The listing builds one solid part. Answer for the finished solid, in the listing's coordinates (mm). Round coordinates to 2 decimals unless told otherwise and drop trailing zeros. Write each loop counter-clockwise with the first axis right and the second up, starting at its lowest first coordinate (ties: lowest second). Pieces come first, ordered by that corner, then holes.
Item 1: Find section C-C on z = -77.5. Give the vertices of the cut face in (x, y) (3 decimals).
Item 2: Find section A-A on x = 0. Give the vertices of the cut face in (y, z), then the cut area to 3 significant figures.
Item 3: Find section B-B on z = 0. Give the vertices of the cut face in (x, y).
Item 4: Find the intervals of material crossed by probe 1 along X at (y, z) = (4.25, -77); probe 2 along X at (y, z) = (0.5, 27); probe 3 along Z at (x, y) = (-22.5, 1.75), in increasing order.
Item 5: Find section D-D on x = 65. Give the vertices of the cut face in (y, z) (3 decimals).
Item 6: For a pull along Z with two mould halves and no side action, classify faces 1 (the face through (-39, 0, -1)), 2 (the face through (-26.063, 3.118, 67.626)), 3 (the face through (-1, 3, 85)) as +Z half, -Z half, draft (parallel to the pull), parting line (faces both ways), or undercut.
```python
from build123d import *

# Parameters (mm, degrees)
SKETCH1_W                      = 170
SKETCH1_H                      = 170
SKETCH1_R                      = 32
BOSS_EXTRUDE3_DEPTH            = 6.35
M4_CLEARANCE_HOLE2_D           = 4.5
M4_CLEARANCE_HOLE2_CSINK_D     = 4.55
M4_CLEARANCE_HOLE2_CSINK_ANGLE = 90
M4_CLEARANCE_HOLE5_D           = 4.5
M4_CLEARANCE_HOLE5_CSINK_D     = 4.55
M4_CLEARANCE_HOLE5_CSINK_ANGLE = 90
M5_CLEARANCE_HOLE1_D           = 5.5
M5_CLEARANCE_HOLE1_CSINK_D     = 5.55
M5_CLEARANCE_HOLE1_CSINK_ANGLE = 90
M5_CLEARANCE_HOLE2_D           = 5.5
M5_CLEARANCE_HOLE2_CSINK_D     = 5.55
M5_CLEARANCE_HOLE2_CSINK_ANGLE = 90


with BuildPart() as part:
    # Sketch1 → Boss-Extrude3 (new body)
    with BuildSketch(Plane(origin=(0, 0, 0), x_dir=(1, 0, 0), z_dir=(0, 1, 0))):
        Rectangle(SKETCH1_W, SKETCH1_H)
        with Locations(Location((0, 0, 0), (0, 0, 270))):
            Circle(SKETCH1_R, mode=Mode.SUBTRACT)
    extrude(amount=BOSS_EXTRUDE3_DEPTH)

    # M4 Clearance Hole2 (through all)
    with Locations(Plane(origin=(0, 0, 0), x_dir=(-1, 0, 0), z_dir=(0, -1, 0))):
        with Locations((-9.188076101, 34.290366833), (25.102290732, 25.102290732), (34.290366833, -9.188076101), (9.188076101, -34.290366833), (-25.102290732, -25.102290732), (-34.290366833, 9.188076101)):
            CounterSinkHole(M4_CLEARANCE_HOLE2_D / 2, M4_CLEARANCE_HOLE2_CSINK_D / 2, counter_sink_angle=M4_CLEARANCE_HOLE2_CSINK_ANGLE)

    # M4 Clearance Hole5 (through all)
    with Locations(Plane(origin=(0, 6.35, 0), x_dir=(1, 0, 0), z_dir=(0, 1, 0))):
        with Locations((-68.301673362, -23.916580707), (-23.916580707, -68.301673362)):
            CounterSinkHole(M4_CLEARANCE_HOLE5_D / 2, M4_CLEARANCE_HOLE5_CSINK_D / 2, counter_sink_angle=M4_CLEARANCE_HOLE5_CSINK_ANGLE)

    # M5 Clearance Hole1 (through all)
    with Locations(Plane(origin=(0, 6.35, 0), x_dir=(1, 0, 0), z_dir=(0, 1, 0))):
        with Locations((-65, -77.5)):
            CounterSinkHole(M5_CLEARANCE_HOLE1_D / 2, M5_CLEARANCE_HOLE1_CSINK_D / 2, counter_sink_angle=M5_CLEARANCE_HOLE1_CSINK_ANGLE)

    # M5 Clearance Hole2 (through all)
    with Locations(Plane(origin=(0, 6.35, 0), x_dir=(1, 0, 0), z_dir=(0, 1, 0))):
        with Locations((-65, 77.5), (65, 77.5), (65, -77.5)):
            CounterSinkHole(M5_CLEARANCE_HOLE2_D / 2, M5_CLEARANCE_HOLE2_CSINK_D / 2, counter_sink_angle=M5_CLEARANCE_HOLE2_CSINK_ANGLE)


solid = part.part
```
Check values:
1. outline: (-85, 0) - (-67.75, 0) - (-67.75, 6.325) - (-67.775, 6.35) - (-85, 6.35) - close; (-62.25, 0) - (62.25, 0) - (62.25, 6.325) - (62.225, 6.35) - (-62.225, 6.35) - (-62.25, 6.325) - close; (67.75, 0) - (85, 0) - (85, 6.35) - (67.775, 6.35) - (67.75, 6.325) - close
2. outline: (0, -85) - (6.35, -85) - (6.35, -32) - (0, -32) - close; (0, 32) - (6.35, 32) - (6.35, 85) - (0, 85) - close
2. area: 673 mm2
3. outline: (-85, 0) - (-32, 0) - (-32, 6.35) - (-85, 6.35) - close; (32, 0) - (85, 0) - (85, 6.35) - (32, 6.35) - close
4. probe 1: x = -85 to -67.7, -62.3 to 62.3, 67.7 to 85
4. probe 2: x = -85 to -17.18, 17.18 to 23.89, 26.31 to 85
4. probe 3: z = -85 to -22.75, 22.75 to 66.55, 70.05 to 85
5. outline: (0, -85) - (6.35, -85) - (6.35, -80.275) - (6.325, -80.25) - (0, -80.25) - close; (0, -74.75) - (6.325, -74.75) - (6.35, -74.725) - (6.35, 74.725) - (6.325, 74.75) - (0, 74.75) - close; (0, 80.25) - (6.325, 80.25) - (6.35, 80.275) - (6.35, 85) - (0, 85) - close
6. face 1: draft
6. face 2: undercut
6. face 3: +Z half
